```python
from build123d import *

# Parameters (mm, degrees)
BOSS_EXTRUDE1_DEPTH = 235
CUT_EXTRUDE1_DEPTH  = 225


with BuildPart() as part:
    # Sketch1 → Boss-Extrude1 (new body)
    with BuildSketch(Plane(origin=(0, 0, 0), x_dir=(1, 0, 0), z_dir=(0, 1, 0))):
        with BuildLine():
            Line((-180, -155), (180, -155))
            ThreePointArc((180, -155), (194.142135624, -149.142135624), (200, -135))
            Line((200, -135), (200, 135))
            ThreePointArc((200, 135), (194.142135624, 149.142135624), (180, 155))
            Line((180, 155), (-180, 155))
            ThreePointArc((-180, 155), (-194.142135624, 149.142135624), (-200, 135))
            Line((-200, 135), (-200, -135))
            ThreePointArc((-200, -135), (-194.142135624, -149.142135624), (-180, -155))
        make_face()
    extrude(amount=BOSS_EXTRUDE1_DEPTH)

    # Sketch2 → Cut-Extrude1 (cut)
    with BuildSketch(Plane(origin=(0, 235, 0), x_dir=(1, 0, 0), z_dir=(0, 1, 0))):
        with BuildLine():
            Line((-180, -142.5), (180, -142.5))
            ThreePointArc((180, -142.5), (187.071067812, -139.571067812), (190, -132.5))
            Line((190, -132.5), (190, 132.5))
            ThreePointArc((190, 132.5), (187.071067812, 139.571067812), (180, 142.5))
            Line((180, 142.5), (-180, 142.5))
            ThreePointArc((-180, 142.5), (-187.071067812, 139.571067812), (-190, 132.5))
            Line((-190, 132.5), (-190, -132.5))
            ThreePointArc((-190, -132.5), (-187.071067812, -139.571067812), (-180, -142.5))
        make_face()
    extrude(amount=-CUT_EXTRUDE1_DEPTH, mode=Mode.SUBTRACT)


solid = part.part
```
Check sheet for the modelled part. Datum: model origin and axes. Units: mm. A direction names the side the tool comes from. Round coordinates to 2 decimals unless told otherwise and drop trailing zeros. Loops run counter-clockwise (first coordinate to the right, second up) from the corner with the lowest first, then second, coordinate; pieces in that order, holes last. Notation, with made-up numbers: (-7.5, 61.5) - (31.5, 61.5) arc R17 ccw to (31.5, 90.5) - close; hole circle Ø1 at (5.5, -2). An arc over 180 degrees is marked (long way). Answer as a JSON object with one key per item and string values. Group by question number.
Q1. Scan lines: line 1 along X through (y, z) = (152, 47); line 2 along Z through (x, y) = (-43.5, 95.5); line 3 along X through (y, z) = (95, -133.5). Record each from-to range of solid material in increasing order. Write a range as [from, to].
Q2. Sectioned sample at B-B, the plane x = -136. Enter the section's corners in (y, z).
Q3. Sectioned sample at A-A, the plane y = 130. Enter the section's corners in (x, z), plus the area to 3 significant figures.
Q4. Set-up check for faces 1 (the face through (-1, 235, 149)), 2 (the face through (190, 124, 2)): record each of +Z, -Z, +X, -X, +Y, -Y from which the full face is reachable in a straight line by a thin tool's end or side.
Q5. Sectioned sample at C-C, the plane z = -69.5. Enter the section's corners in (x, y).
Q6. Gauge pin test, flat end, axial feed: P1, Ø5, axis at x = -58.5, z = 68.5, coming from the +Y side. Record the tip position at first contact, or that the pin passes through.
Q7. Mould release check, pull along Z, two halves, no side actions. Record for faces 3 (the face through (3, 116, -155)), 4 (the face through (-200, 116, -2)), 5 (the face through (-3, 10, -2)): released by +Z, released by -Z, zero draft, split by the parting line, or undercut.
Solution:
{
 "1": {"line 1": "x = [-200, -190], [190, 200]", "line 2": "z = [-155, -142.5], [142.5, 155]", "line 3": "x = [-200, -189.95], [189.95, 200]"},
 "2": {"outline": "(0, -155) - (235, -155) - (235, -142.5) - (10, -142.5) - (10, 142.5) - (235, 142.5) - (235, 155) - (0, 155) - close"},
 "3": {"outline": "(-200, -135) arc R20 ccw to (-180, -155) - (180, -155) arc R20 ccw to (200, -135) - (200, 135) arc R20 ccw to (180, 155) - (-180, 155) arc R20 ccw to (-200, 135) - close; hole (-190, -132.5) arc R10 ccw to (-180, -142.5) - (180, -142.5) arc R10 ccw to (190, -132.5) - (190, 132.5) arc R10 ccw to (180, 142.5) - (-180, 142.5) arc R10 ccw to (-190, 132.5) - close", "area": "15,400 mm²"},
 "4": {"face 1": "+Z, -Z, +X, -X, +Y", "face 2": "+Y"},
 "5": {"outline": "(-200, 0) - (200, 0) - (200, 235) - (190, 235) - (190, 10) - (-190, 10) - (-190, 235) - (-200, 235) - close"},
 "6": {"P1": "stops at y = 10"},
 "7": {"face 3": "released by -Z", "face 4": "zero draft", "face 5": "undercut"}
}
